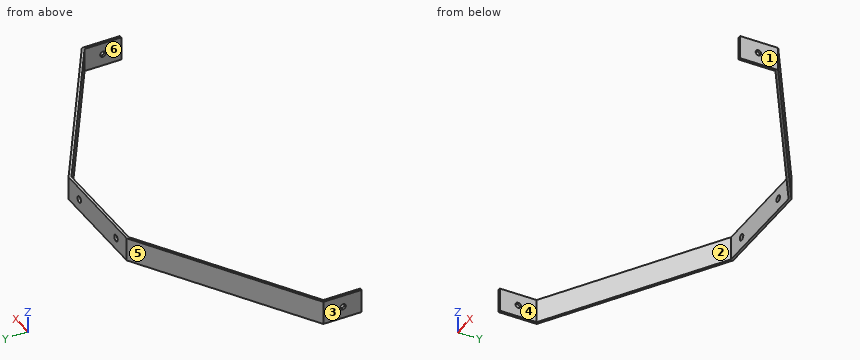
Autodesk Inventor part; units mm, degrees
ref_plane "YZ Plane" through (0, 0, 0) normal (1, 0, 0) x (0, 1, 0)
ref_plane "XZ Plane" through (0, 0, 0) normal (0, 1, 0) x (-1, 0, 0)
ref_plane "XY Plane" through (0, 0, 0) normal (0, 0, 1) x (1, 0, 0)
sketch "Sketch1" plane through (0, 0, 0) normal (0, 0, 1) x (1, 0, 0)
  line L0 (0, 0) -> (-1.35, 0)
  line L1 (0, 0) -> (0, 20)
  line L2 (0, 20) -> (90.49, 20) construction
  line L3 (90.49, 20) -> (90.49, 76.5) construction
  line L4 (90.49, 76.5) -> (0, 20)
  line L5 (90.49, 76.5) -> (147.79, 76.5)
  line L6 (119.14, 76.5) -> (119.14, 94.3884) construction
  line L7 (-1.35, 0) -> (-1.35, 20.7486)
  line L8 (-1.35, 20.7486) -> (90.1032, 77.85)
  line L9 (119.14, 77.85) -> (90.1032, 77.85)
  line L10 (238.28, 0) -> (239.63, 0)
  line L11 (238.28, 0) -> (238.28, 20)
  line L12 (147.79, 76.5) -> (238.28, 20)
  line L13 (147.79, 76.5) -> (90.49, 76.5)
  line L14 (239.63, 0) -> (239.63, 20.7486)
  line L15 (239.63, 20.7486) -> (148.1768, 77.85)
  line L16 (119.14, 77.85) -> (148.1768, 77.85)
  dimension "d0" = 1.35
  dimension "d1" = 20
  dimension "d2" = 90.49
  dimension "d3" = 56.5
  dimension "d4" = 57.3
  dimension "d5" = 1.35
  dimension "d6" = 1.35
extrude "Extrusion1" add sketch "Sketch1" along normal mid plane 12.9
sketch "Sketch2" plane through (90.1032, 77.85, 6.45) normal (0, 1, 0) x (1, 0, 0)
  circle A0 centre (10.7168, 6.45) radius 1.75
  line L0 (10.7168, 6.45) -> (47.3568, 6.45)
  circle A1 centre (47.3568, 6.45) radius 1.75
  line L1 (0, 12.9) -> (58.0737, 12.9)
  point P0 (-90.1032, 6.45)
  point P1 (29.0368, 12.9)
  point P2 (29.0368, 6.45)
  dimension "d9" = 3.5
  dimension "d10" = 36.64
  dimension "d11" = 3.5
  dimension "d12" = 0
extrude "Extrusion2" cut sketch "Sketch2" against normal blind 12.9
sketch "Sketch4" plane through (239.63, 0, 6.45) normal (1, 0, 0) x (0, 0, -1)
  circle A0 centre (6.45, 10) radius 1.5
  point P0 (6.45, 0)
  dimension "d15" = 3
extrude "Extrusion3" cut sketch "Sketch4" against normal through all
properties part number "A-MainGear"
Part model, mm, in its own coordinate system. Face numbers are marked on the shaded views. A direction names the side the tool comes from. Coordinates: 2 decimals unless noted, no trailing zeros. Order: outer loops, then holes, each group sorted by start corner. A loop starts at its lowest first (then second) coordinate and runs counter-clockwise, first axis right, second up.
(1) Slice it at C-C, the plane x = 173. Write the cut outline in (y, z).
Check sheet entries:
outline: (60.76, -6.45) - (62.35, -6.45) - (62.35, 6.45) - (60.76, 6.45) - close
(2) Probe L1, parallel to X at y = 9.5, z = -4.5; L2, parallel to Z at x = 137.46, y = 77.6; L3, parallel to X at y = 77.2, z = 0. List the from-to ranges inside material, lowest first.
Check sheet entries:
L1: x = -1.35 to 0, 238.28 to 239.63
L2: z = -6.45 to -1.75, 1.75 to 6.45
L3: x = 89.06 to 99.07, 102.57 to 135.71, 139.21 to 149.22
(3) Slice it at A-A, the plane z = -4. Write the cut outline in (x, y).
Check sheet entries:
outline: (-1.35, 0) - (0, 0) - (0, 20) - (90.49, 76.5) - (147.79, 76.5) - (238.28, 20) - (238.28, 0) - (239.63, 0) - (239.63, 20.75) - (148.18, 77.85) - (90.1, 77.85) - (-1.35, 20.75) - close
(4) Pin check, flat tips, straight feed: pin 1 Ø2.5 at (y, z) = (10, 0) entering from +X; pin 2 Ø6 at (y, z) = (24.5, 3) entering from +X; pin 3 Ø2 at (y, z) = (51.5, -2.5) entering from -X; pin 4 Ø1.5 at (x, z) = (30.5, 5) entering from -Y. Stop position of each tip, or through.
Check sheet entries:
pin 1: passes through
pin 2: stops at x = 238.43
pin 3: stops at x = 46.3
pin 4: stops at y = 38.58
(5) Pull direction X, two halves, no side cores. Call the marked faces 1, 2, 3 and 4: pulls with the +X half, pulls with the -X half, needs draft (parallel to the pull), parting line crosses it, or undercut.
Check sheet entries:
face 1: pulls with the +X half
face 2: undercut
face 3: pulls with the -X half
face 4: undercut
(6) Tool access for the marked faces 5 and 6: list every direction of +Z, -Z, +X, -X, +Y, -Y with a clear straight run to the whole face (end or side of a thin tool).
Check sheet entries:
face 5: +Z, -Z, -X, +Y
face 6: +Z, -Z, -Y
(7) Slice it at B-B, the plane y = 43.5. Write the cut outline in (x, z), and give its area (3 significant figures).
Check sheet entries:
outline: (35.09, -6.45) - (37.64, -6.45) - (37.64, 6.45) - (35.09, 6.45) - close; (200.64, -6.45) - (203.19, -6.45) - (203.19, 6.45) - (200.64, 6.45) - close
area: 65.8 mm2
